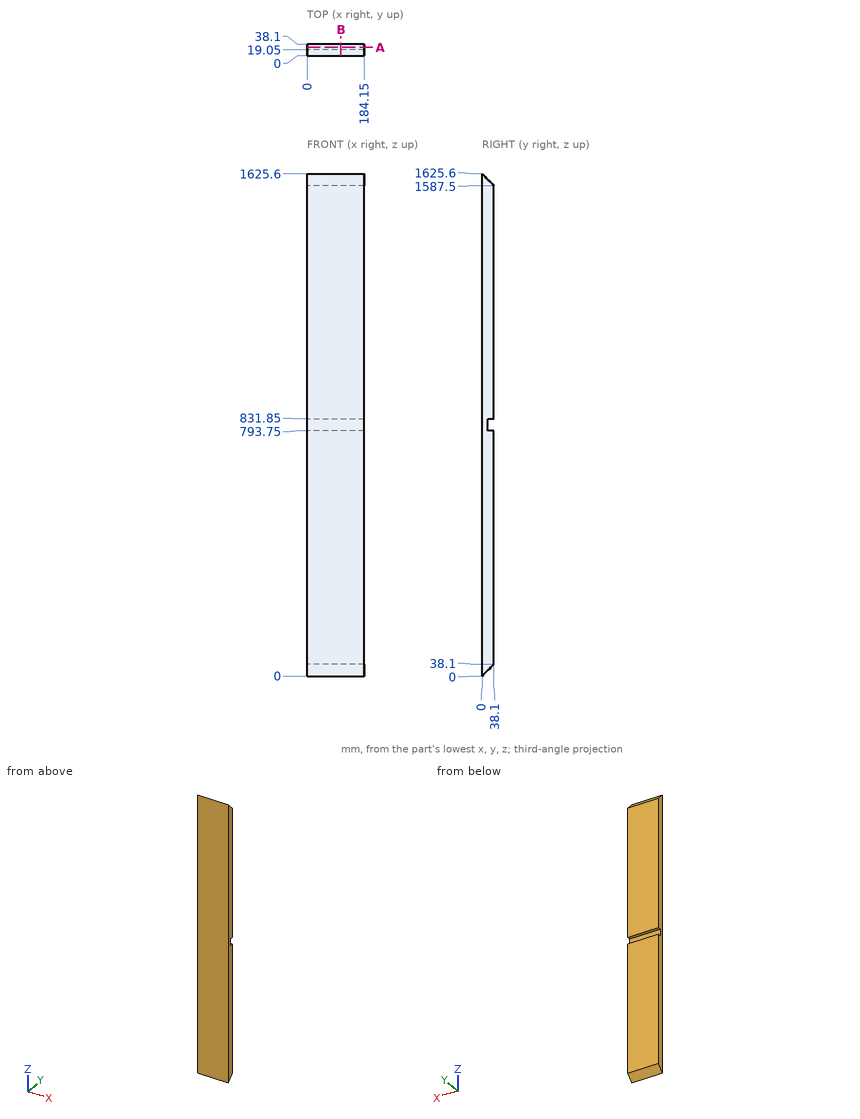
Check sheet for the drawn part. Datum: minimum x, y, z corner. Units: mm. Round coordinates to 2 decimals unless told otherwise and drop trailing zeros. Order: outer loops, then holes, each group sorted by start corner. A loop starts at its lowest first (then second) coordinate and runs counter-clockwise, first axis right, second up.
1) Go/stop test with flat-tipped pins: pin 1 Ø19 at (x, z) = (117.5, 806) entering from +Y; pin 2 Ø9.5 at (x, y) = (115, 29.5) entering from -Z; pin 3 Ø8 at (x, y) = (158, 31.5) entering from +Z. Record where each tip stops, or that it passes through.
2) Section check B-B (x = 109). Record the boundary of the cut face in (y, z), and give its area (3 significant figures).
3) Scan lines: line 1 (Z direction, x = 64.5, y = 31.5); line 2 (Z direction, x = 98.5, y = 23.5); line 3 (Y direction, x = 126.5, z = 803). Record each from-to range of solid material in increasing order.
4) Section check A-A (y = 27). Record the boundary of the cut face in (x, z).
Result:
1. pin 1: stops at y = 19.05
1. pin 2: stops at z = 24.75
1. pin 3: stops at z = 1598.1
2. outline: (0, 0) - (38.1, 38.1) - (38.1, 793.75) - (19.05, 793.75) - (19.05, 831.85) - (38.1, 831.85) - (38.1, 1587.5) - (0, 1625.6) - close
2. area: 59,800 mm2
3. line 1: z = 31.5 to 793.75, 831.85 to 1594.1
3. line 2: z = 23.5 to 793.75, 831.85 to 1602.1
3. line 3: y = 0 to 19.05
4. outline: (0, 27) - (184.15, 27) - (184.15, 793.75) - (0, 793.75) - close; (0, 831.85) - (184.15, 831.85) - (184.15, 1598.6) - (0, 1598.6) - close
